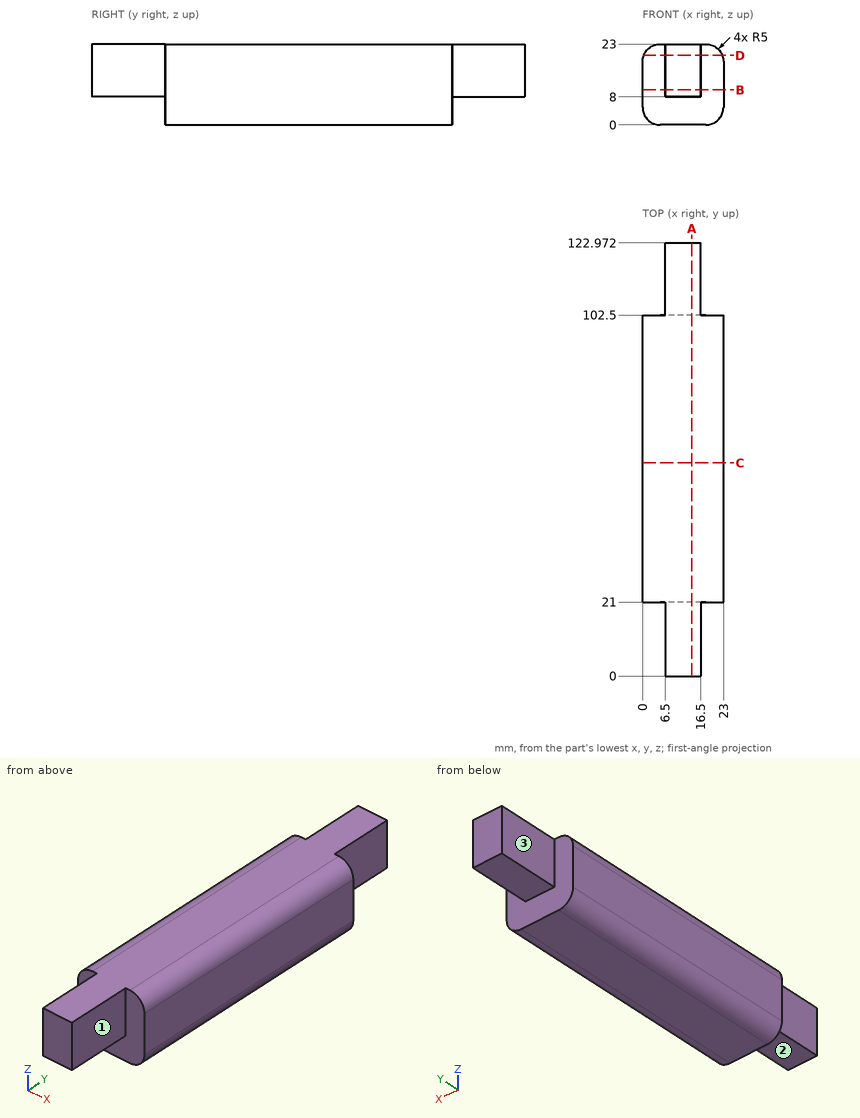
Source: three-view drawing plus pictorial views. Frame: mm from the lowest corner of the part. A direction names the side the tool comes from. Round coordinates to 2 decimals unless told otherwise and drop trailing zeros. Order: outer loops, then holes, each group sorted by start corner. A loop starts at its lowest first (then second) coordinate and runs counter-clockwise, first axis right, second up. Notation, with made-up numbers: (-9, 2) -> (10, 2) arc R15 ccw to (10, 9) -> close; hole circle Ø3 at (88, 81). An arc over 180 degrees is marked (long way). Use one line per item in the form item = value.
(1) Section C-C on y = 60.5. Return loops of the section in (x, z).
Results list:
outline = (0, 5) arc R5 ccw to (5, 0) -> (18, 0) arc R5 ccw to (23, 5) -> (23, 18) arc R5 ccw to (18, 23) -> (5, 23) arc R5 ccw to (0, 18) -> close
(2) Section A-A on x = 14. Return loops of the section in (y, z).
Results list:
outline = (0, 8) -> (21, 8) -> (21, 0) -> (102.5, 0) -> (102.5, 8) -> (122.97, 8) -> (122.97, 23) -> (0, 23) -> close
(3) First-contact query: pin 1 Ø7.5 at (y, z) = (117.5, 15.5) entering from -X; pin 2 Ø8 at (x, y) = (11.5, 110) entering from -Z; pin 3 Ø4.5 at (y, z) = (108.5, 18.5) entering from +X. Flat tips, straight axial feed; report the tip coordinate or a pass-through.
Results list:
pin_1 = 6.5
pin_2 = 8
pin_3 = 16.5
(4) Section D-D on z = 19.75. Return loops of the section in (x, y).
Results list:
outline = (0.32, 21) -> (6.5, 21) -> (6.5, 0) -> (16.5, 0) -> (16.5, 21) -> (22.68, 21) -> (22.68, 102.5) -> (16.5, 102.5) -> (16.5, 122.97) -> (6.5, 122.97) -> (6.5, 102.5) -> (0.32, 102.5) -> close
(5) Ray query, probe 1 along X at (y, z) = (106, 10.5); probe 2 along Y at (x, z) = (16.25, 6.75); probe 3 along Z at (x, y) = (6.75, 108). Return the intervals inside material, ascending. Write a range as [from, to].
Results list:
probe_1 = [6.5, 16.5]
probe_2 = [21, 102.5]
probe_3 = [8, 23]
(6) Section B-B on z = 10. Return loops of the section in (x, y).
Results list:
outline = (0, 21) -> (6.5, 21) -> (6.5, 0) -> (16.5, 0) -> (16.5, 21) -> (23, 21) -> (23, 102.5) -> (16.5, 102.5) -> (16.5, 122.97) -> (6.5, 122.97) -> (6.5, 102.5) -> (0, 102.5) -> close
(7) Access query for the marked faces 1, 2 and 3. Directions: +Z, -Z, +X, -X, +Y, -Y. A direction counts if a zero-diameter tool reaches every point of the face in a straight line with its end or side. Return the directions, or none.
Results list:
face_1 = +Z, -Z, +X, -Y
face_2 = -Z, +X, -X, -Y
face_3 = +Z, -Z, -X, +Y
